from build123d import *

# Parameters (mm, degrees)
BOSS_EXTRUDE1_START       = -4
BOSS_EXTRUDE1_OUTLINE_R   = 2.2
BOSS_EXTRUDE1_OUTLINE_R_2 = 1.025
BOSS_EXTRUDE1_OUTLINE_R_3 = 6.575
BOSS_EXTRUDE1_DEPTH       = 4
SKETCH3_R                 = 8.875
SKETCH3_R_2               = 7.075
CUT_EXTRUDE1_DEPTH        = 1.05
BOSS_EXTRUDE2_START       = -4
SKETCH4_R                 = 1.025
BOSS_EXTRUDE2_DEPTH       = 0.75
FILLET1_R                 = 1
BOSS_EXTRUDE3_START       = -5
SKETCH5_R                 = 32.5
SKETCH5_R_2               = 1.025
SKETCH5_R_3               = 8.875
BOSS_EXTRUDE3_DEPTH       = 5
SKETCH6_R                 = 2.2
CUT_EXTRUDE2_DEPTH        = 5
SKETCH7_R                 = 20.6
SKETCH7_R_2               = 15.6
CUT_EXTRUDE3_DEPTH        = 2.5
BOSS_EXTRUDE4_START       = 1
SKETCH8_R                 = 1.025
BOSS_EXTRUDE4_DEPTH       = 1


# Read off the part's stored shape, not the designer's step: Boss-Extrude1
with BuildPart() as part:
    # Boss-Extrude1 outline → Boss-Extrude1 (new body)
    with BuildSketch(Plane.XY.offset(BOSS_EXTRUDE1_START)):
        with BuildLine():
            Line((-5.8, 12.8), (-5.8, -12.8))
            ThreePointArc((-5.8, -12.8), (-1.992388155, -21.992388155), (7.2, -25.8))
            Line((7.2, -25.8), (32.8, -25.8))
            ThreePointArc((32.8, -25.8), (41.992388155, -21.992388155), (45.8, -12.8))
            Line((45.8, -12.8), (45.8, 12.8))
            ThreePointArc((45.8, 12.8), (41.992388155, 21.992388155), (32.8, 25.8))
            Line((32.8, 25.8), (7.2, 25.8))
            ThreePointArc((7.2, 25.8), (-1.992388155, 21.992388155), (-5.8, 12.8))
        make_face()
        with Locations((25, -22)):
            Circle(BOSS_EXTRUDE1_OUTLINE_R, mode=Mode.SUBTRACT)
        with Locations((20, -11.1252)):
            Circle(BOSS_EXTRUDE1_OUTLINE_R_2, mode=Mode.SUBTRACT)
        with Locations((-2, 0)):
            Circle(BOSS_EXTRUDE1_OUTLINE_R, mode=Mode.SUBTRACT)
        with Locations((20, 0)):
            Circle(BOSS_EXTRUDE1_OUTLINE_R_3, mode=Mode.SUBTRACT)
        with Locations((20, 11.1252)):
            Circle(BOSS_EXTRUDE1_OUTLINE_R_2, mode=Mode.SUBTRACT)
        with Locations((42, 0)):
            Circle(BOSS_EXTRUDE1_OUTLINE_R, mode=Mode.SUBTRACT)
        with Locations((25, 22)):
            Circle(BOSS_EXTRUDE1_OUTLINE_R, mode=Mode.SUBTRACT)
    extrude(amount=BOSS_EXTRUDE1_DEPTH)

    # Sketch3 → Cut-Extrude1 (cut)
    with BuildSketch(Plane.XY):
        with Locations((20, 0)):
            Circle(SKETCH3_R)
        with Locations((20, 0)):
            Circle(SKETCH3_R_2, mode=Mode.SUBTRACT)
    extrude(amount=-CUT_EXTRUDE1_DEPTH, mode=Mode.SUBTRACT)

    # Sketch4 → Boss-Extrude2 (add)
    with BuildSketch(Plane.XY.offset(BOSS_EXTRUDE2_START)):
        with Locations((20, 11.1252)):
            Circle(SKETCH4_R)
        with Locations((20, -11.1252)):
            Circle(SKETCH4_R)
    extrude(amount=BOSS_EXTRUDE2_DEPTH)

    # Fillet1
    fillet1_edges = [part.edges().sort_by_distance(p)[0] for p in [
        (18.975, 11.1252, -3.25),
        (18.975, -11.1252, -3.25),
    ]]
    fillet(fillet1_edges, radius=FILLET1_R)

    # Sketch5 → Boss-Extrude3 (add)
    with BuildSketch(Plane.XY.offset(BOSS_EXTRUDE3_START)):
        with Locations((20, 0)):
            Circle(SKETCH5_R)
        with Locations((20, -11.1252)):
            Circle(SKETCH5_R_2, mode=Mode.SUBTRACT)
        with Locations((20, 11.1252)):
            Circle(SKETCH5_R_2, mode=Mode.SUBTRACT)
        with Locations((20, 0)):
            Circle(SKETCH5_R_3, mode=Mode.SUBTRACT)
    extrude(amount=BOSS_EXTRUDE3_DEPTH)

    # Sketch6 → Cut-Extrude2 (cut)
    with BuildSketch(Plane.XY):
        with Locations((-8.496265533, -0.461357402)):
            Circle(SKETCH6_R)
        with Locations((20, 28.5)):
            Circle(SKETCH6_R)
        with Locations((48.496265533, -0.461357402)):
            Circle(SKETCH6_R)
        with Locations((20, -28.5)):
            Circle(SKETCH6_R)
    extrude(amount=-CUT_EXTRUDE2_DEPTH, mode=Mode.SUBTRACT)

    # Sketch7 → Cut-Extrude3 (cut)
    with BuildSketch(Plane(origin=(0, 0, -5), x_dir=(-1, 0, 0), z_dir=(0, 0, -1))):
        with Locations((-20, 0)):
            Circle(SKETCH7_R)
        with Locations((-20, 0)):
            Circle(SKETCH7_R_2, mode=Mode.SUBTRACT)
    extrude(amount=-CUT_EXTRUDE3_DEPTH, mode=Mode.SUBTRACT)

    # Sketch8 → Boss-Extrude4 (add)
    with BuildSketch(Plane(origin=(0, 0, -4), x_dir=(-1, 0, 0), z_dir=(0, 0, -1)).offset(BOSS_EXTRUDE4_START)):
        with Locations(Location((-20, -11.1252, 0), (0, 0, 180))):
            Circle(SKETCH8_R)
        with Locations(Location((-20, 11.1252, 0), (0, 0, 180))):
            Circle(SKETCH8_R)
    extrude(amount=-BOSS_EXTRUDE4_DEPTH)


solid = part.part
Can you work these out from the model? Positions are in its coordinate system, mm. A direction names the side the tool comes from. Coordinates: 2 decimals unless noted, no trailing zeros. Order: outer loops, then holes, each group sorted by start corner. A loop starts at its lowest first (then second) coordinate and runs counter-clockwise, first axis right, second up. Notation, with made-up numbers: M 52.5,12 L 93.5,12 A30 cw 93.5,36 Z; hole C 51,14.5 d11. An arc over 180 degrees is marked long. Answer as CSV lines item,"result".
(1) If we mould it in two halves opening along X, with no side actions, what happens to faces 1 (the flat face through (13, 0, -4)), 2 (the cylindrical face through (-3.95, 21.97, -2.54)), 3 (the flat face through (41, 0, -5))? For each: released by +X, released by -X, zero draft, split by the parting line, or undercut.
Geometry check:
face 1,"undercut"
face 2,"split by the parting line"
face 3,"zero draft"
(2) Please list where these lines run through material, in increasing order: L1, parallel to Y at x = 20, z = -1.7 (3 decimals); L2, parallel to X at y = -9, z = -2.8; L3, parallel to Y at x = 21, z = -4.6.
Geometry check:
L1,"-32.5 to -30.7, -26.3 to -12.15, -10.1 to -6.575, 6.575 to 10.1, 12.15 to 26.3, 30.7 to 32.5"
L2,"-11.23 to 1.47, 7.26 to 32.74, 38.53 to 51.23"
L3,"-32.48 to -30.46, -26.54 to -20.58, -15.57 to -8.82, 8.82 to 15.57, 20.58 to 26.54, 30.46 to 32.48"
(3) I'm going to push flat-ended pins straight in: pin 1 (21 mm diameter, centred on x = 20, y = 0, fed in from -Z); pin 2 (1.5 mm diameter, centred on x = 29, z = -0.5, fed in from -Y). Where does each tip first touch, or does it pass through?
Geometry check:
pin 1,"z = -5"
pin 2,"y = -31.44"
(4) Suppose I cut it at A-A on x = 17. Please give me the cut outline in (y, z).
Geometry check:
outline,"M -32.36,-5 L -20.38,-5 L -20.38,-2.5 L -15.31,-2.5 L -15.31,-5 L -8.35,-5 L -8.35,-4 L -5.85,-4 L -5.85,0 L -6.41,0 L -6.41,-1.05 L -8.35,-1.05 L -8.35,0 L -32.36,0 Z; M 5.85,-4 L 8.35,-4 L 8.35,-5 L 15.31,-5 L 15.31,-2.5 L 20.38,-2.5 L 20.38,-5 L 32.36,-5 L 32.36,0 L 8.35,0 L 8.35,-1.05 L 6.41,-1.05 L 6.41,0 L 5.85,0 Z"
(5) Suppose I cut it at B-B on y = 4.5. Please give me the cut outline in (x, z).
Geometry check:
outline,"M -12.19,-5 L -0.1,-5 L -0.1,-2.5 L 5.06,-2.5 L 5.06,-5 L 12.35,-5 L 12.35,-4 L 15.21,-4 L 15.21,0 L 14.54,0 L 14.54,-1.05 L 12.35,-1.05 L 12.35,0 L -12.19,0 Z; M 24.79,-4 L 27.65,-4 L 27.65,-5 L 34.94,-5 L 34.94,-2.5 L 40.1,-2.5 L 40.1,-5 L 52.19,-5 L 52.19,0 L 27.65,0 L 27.65,-1.05 L 25.46,-1.05 L 25.46,0 L 24.79,0 Z"
(6) On a 3-axis mill with a long thin cutter (end or side, diameter ignored), from which of +Z, -Z, +X, -X, +Y, -Y can I reach the whole of each face in a straight line? I mean faces 4 (the flat face through (27, 7, -5)), 5 (the cylindrical face through (19.245, 11.818, -1.141)), 6 (the flat face through (12, 14, -2.5)). Say none if no direction works.
Geometry check:
face 4,"-Z, +X, -X, +Y, -Y"
face 5,"+Z"
face 6,"-Z"
(7) Suppose I cut it at D-D on y = -28.5. Please give me the cut outline in (x, z).
Geometry check:
outline,"M 4.38,-5 L 17.8,-5 L 17.8,0 L 4.38,0 Z; M 22.2,-5 L 35.62,-5 L 35.62,0 L 22.2,0 Z"
(8) Suppose I cut it at C-C on x = 32.5. Please give me the cut outline in (y, z), plus the area to 3 significant figures.
Geometry check:
outline,"M -30,-5 L -16.37,-5 L -16.37,-2.5 L -9.33,-2.5 L -9.33,-5 L 9.33,-5 L 9.33,-2.5 L 16.37,-2.5 L 16.37,-5 L 30,-5 L 30,0 L -30,0 Z"
area,"265 mm^2"
